Here's the drawing with two shaded views (mm, measured from the low corner). I have some questions. Coordinates: 2 decimals unless noted, no trailing zeros. Loops run counter-clockwise (first coordinate to the right, second up) from the corner with the lowest first, then second, coordinate; pieces in that order, holes last. Notation, with made-up numbers: (77.25, 16.25) - (104.25, 16.25) arc R23 cw to (104.25, 28.25) - close; hole circle Ø1 at (43, 34). An arc over 180 degrees is marked (long way). Use a Markdown table: item, result.
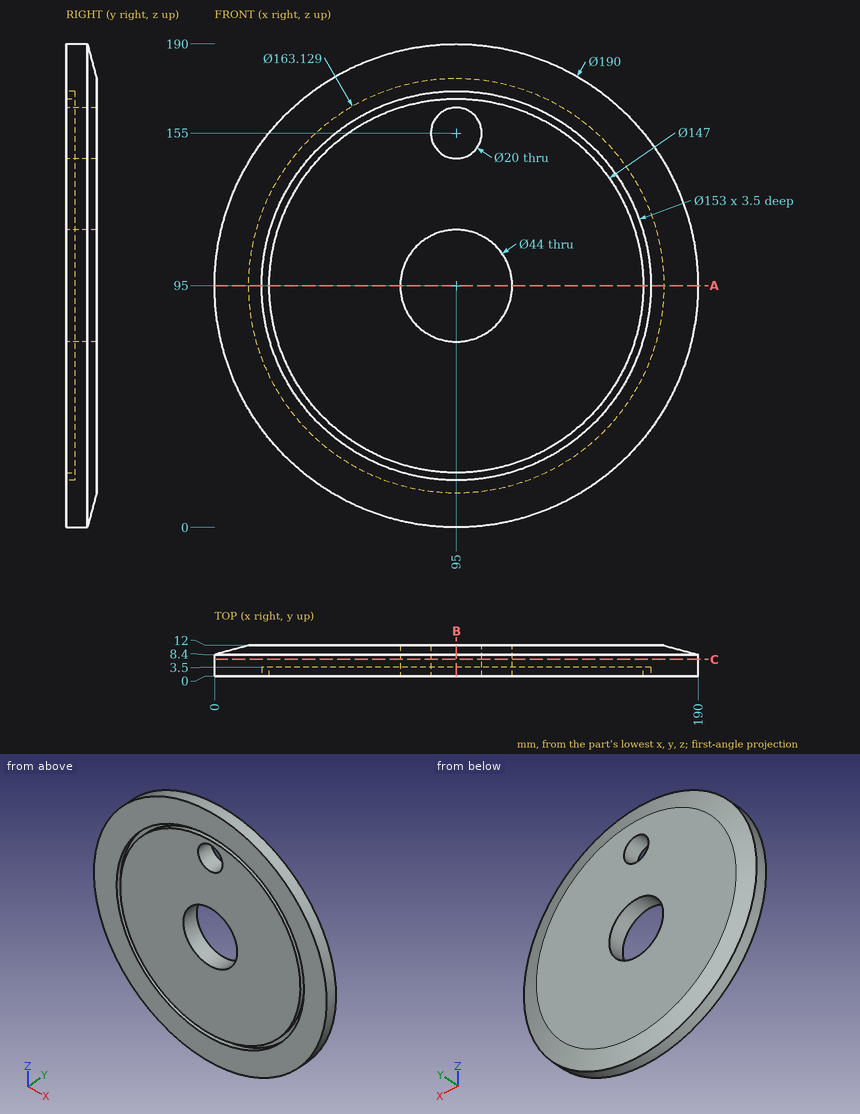
Q1. I want a section at C-C, the plane y = 6.5. Write out the boundary of the cut face in (x, z), then the cut area to 3 significant figures.
Check values:
| item | result |
|---|---|
| outline | circle Ø190 at (95, 95); hole circle Ø44 at (95, 95); hole circle Ø20 at (95, 155) |
| area | 26,500 mm^2 |
Q2. Please list where these lines run through material, in increasing order: L1, parallel to Z at x = 33.5, y = 3; L2, parallel to Y at x = 80, z = 168; L3, parallel to X at y = 3, z = 41.5. Write a range as from..to.
Check values:
| item | result |
|---|---|
| L1 | 22.59..49.5, 54.75..135.25, 140.5..167.41 |
| L2 | 3.5..12 |
| L3 | 16.5..40.32, 44.6..145.4, 149.68..173.5 |
Q3. I want a section at A-A, the plane z = 95. Write out the boundary of the cut face in (x, y) (1 decimal).
Check values:
| item | result |
|---|---|
| outline | (0, 0) - (18.5, 0) - (18.5, 3.5) - (21.5, 3.5) - (21.5, 0) - (73, 0) - (73, 12) - (13.4, 12) - (0, 8.4) - close; (117, 0) - (168.5, 0) - (168.5, 3.5) - (171.5, 3.5) - (171.5, 0) - (190, 0) - (190, 8.4) - (176.6, 12) - (117, 12) - close |
Q4. Will these pins go through, and if not, where does the flat tip stop? P1, Ø5, axis at x = 62.5, y = 2, coming from the -Z side; P2, Ø5, axis at x = 112, y = 9, coming from the +Z side; P3, Ø16, axis at x = 95, z = 155, coming from the +Y side; P4, Ø1.5, axis at x = 129.5, z = 20, coming from the +Y side.
Check values:
| item | result |
|---|---|
| P1 | z = 4.86 |
| P2 | z = 188.88 |
| P3 | through |
| P4 | y = 11.94 |
Q5. I want a section at B-B, the plane x = 95. Write out the boundary of the cut face in (y, z) (1 decimal), then the cut area to 3 significant figures.
Check values:
| item | result |
|---|---|
| outline | (0, 0) - (8.4, 0) - (12, 13.4) - (12, 73) - (0, 73) - (0, 21.5) - (3.5, 21.5) - (3.5, 18.5) - (0, 18.5) - close; (0, 117) - (12, 117) - (12, 145) - (0, 145) - close; (0, 165) - (12, 165) - (12, 176.6) - (8.4, 190) - (0, 190) - (0, 171.5) - (3.5, 171.5) - (3.5, 168.5) - (0, 168.5) - close |
| area | 1,440 mm^2 |
